from build123d import *

# Parameters (mm, degrees)
F0_R     = 8
F1_DEPTH = 5
F2_R     = 4
F3_DEPTH = 99.8
F4_R     = 1


with BuildPart() as f1:
    # F0 (on Top) → F1 (new body)
    with BuildSketch(Plane.XY):
        Circle(F0_R)
    extrude(amount=F1_DEPTH)

    # F2 (on face) → F3 (join)
    with BuildSketch(Plane(origin=(0, 0, 0), x_dir=(1, 0, 0), z_dir=(0, 0, -1))):
        Circle(F2_R)
    extrude(amount=F3_DEPTH)

    # F4
    f4_edges = [f1.edges().sort_by_distance(p)[0] for p in [
        (-4, 0, -99.8),
        (-8, 0, 0),
        (-8, 0, 5),
    ]]
    fillet(f4_edges, radius=F4_R)


solid = f1.part
Read the model definition and answer for the solid it produces. Units are mm, in the model's axes. A direction names the side the tool comes from. Coordinates: 2 decimals unless noted, no trailing zeros. Loops run counter-clockwise (first coordinate to the right, second up) from the corner with the lowest first, then second, coordinate; pieces in that order, holes last.
Q1. Which of the six approach directions +Z, -Z, +X, -X, +Y, -Y give full straight-line access (tool end or side, diameter ignored) to faces 1 (the face through (3, -3, 0)), 2 (the face through (-1.73, -7.81, 2.48))?
Q2. The part is cut by section C-C on z = -72.5. Write down the section's boundary in (x, y), and give its area (3 significant figures).
Q3. Each of these flat-tipped pins is pushed along its axis until it touches: pin 1 Ø2 at (x, z) = (3, -27.5) entering from -Y; pin 2 Ø6 at (y, z) = (1, -13.5) entering from -X; pin 3 Ø3 at (x, z) = (-0.5, -20) entering from -Y. Where does it stop, or does it pass through?
Q4. The part is cut by section A-A on y = 0. Write down the section's boundary in (x, z), and give its area (3 significant figures).
Q5. Consider probe 1 along Z at (x, y) = (-5.25, 2.25); probe 2 along Y at (x, z) = (0.25, -6.5); probe 3 along Y at (x, z) = (1.25, -44.5). Determine where each line is inside the solid, lowest interval first.
Results below:
1. face 1: -Z
1. face 2: +Z, -Z
2. outline: circle Ø8 at (0, 0)
2. area: 50.3 mm2
3. pin 1: stops at y = -3.46
3. pin 2: stops at x = -4
3. pin 3: stops at y = -4
4. outline: (-8, 1) arc R1 ccw to (-7, 0) - (-4, 0) - (-4, -98.8) arc R1 ccw to (-3, -99.8) - (3, -99.8) arc R1 ccw to (4, -98.8) - (4, 0) - (7, 0) arc R1 ccw to (8, 1) - (8, 4) arc R1 ccw to (7, 5) - (-7, 5) arc R1 ccw to (-8, 4) - close
4. area: 877 mm2
5. probe 1: z = 0 to 5
5. probe 2: y = -3.99 to 3.99
5. probe 3: y = -3.8 to 3.8
